from build123d import *

# Parameters (mm, degrees)
SKETCH1_R                           = 5
BOSS_EXTRUDE1_DEPTH                 = 403.4811
CHAMFER1_SIZE                       = 0.5
M5X0_8_TAPPED_HOLE1_D               = 4.2
M5X0_8_TAPPED_HOLE1_DEPTH           = 16.4
M5X0_8_TAPPED_HOLE1_TIP             = 1.2618073
M5X0_8_TAPPED_HOLE1_ON_FACE_2_D     = 4.2
M5X0_8_TAPPED_HOLE1_ON_FACE_2_DEPTH = 16.4
M5X0_8_TAPPED_HOLE1_ON_FACE_2_TIP   = 1.2618073


with BuildPart() as part:
    # Sketch1 → Boss-Extrude1 (new body)
    with BuildSketch(Plane.XY):
        Circle(SKETCH1_R)
    extrude(amount=BOSS_EXTRUDE1_DEPTH)

    # Chamfer1
    chamfer1_edges = [part.edges().sort_by_distance(p)[0] for p in [
        (-5, 0, 0),
        (-5, 0, 403.4811),
    ]]
    chamfer(chamfer1_edges, length=CHAMFER1_SIZE)

    # M5x0.8 Tapped Hole1
    with Locations(Plane.XY.offset(403.4811)):
        with Locations((0, 0)):
            Hole(M5X0_8_TAPPED_HOLE1_D / 2, depth=M5X0_8_TAPPED_HOLE1_DEPTH)
            with Locations((0, 0, -(M5X0_8_TAPPED_HOLE1_DEPTH + M5X0_8_TAPPED_HOLE1_TIP / 2))):  # 118° drill point
                Cone(0, M5X0_8_TAPPED_HOLE1_D / 2, M5X0_8_TAPPED_HOLE1_TIP, mode=Mode.SUBTRACT)

    # M5x0.8 Tapped Hole1 on face 2
    with Locations(Plane(origin=(0, 0, 0), x_dir=(-1, 0, 0), z_dir=(0, 0, -1))):
        with Locations((0, 0)):
            Hole(M5X0_8_TAPPED_HOLE1_ON_FACE_2_D / 2, depth=M5X0_8_TAPPED_HOLE1_ON_FACE_2_DEPTH)
            with Locations((0, 0, -(M5X0_8_TAPPED_HOLE1_ON_FACE_2_DEPTH + M5X0_8_TAPPED_HOLE1_ON_FACE_2_TIP / 2))):  # 118° drill point
                Cone(0, M5X0_8_TAPPED_HOLE1_ON_FACE_2_D / 2, M5X0_8_TAPPED_HOLE1_ON_FACE_2_TIP, mode=Mode.SUBTRACT)


solid = part.part
Geometry: final body of the model. Coordinates: model frame, mm. Give positions to 0.01 mm unless a question says otherwise; leave off trailing zeros. Order: outer loops, then holes, each group sorted by start corner. A loop starts at its lowest first (then second) coordinate and runs counter-clockwise, first axis right, second up. Notation, with made-up numbers: (59.5, 87.25) -> (108.5, 87.25) arc R22 ccw to (108.5, 96.25) -> close; hole circle Ø6 at (65.5, 10.5). An arc over 180 degrees is marked (long way). Answer as a JSON object with one key per item and string values.
Q1. Material intervals for probe 1 along Y at (x, z) = (0, 7.25); probe 2 along Y at (x, z) = (-0.25, 210); probe 3 along X at (y, z) = (-0.5, 143), sorted ascending.
Entries:
{"probe 1": "y = -5 to -2.1, 2.1 to 5", "probe 2": "y = -4.99 to 4.99", "probe 3": "x = -4.97 to 4.97"}
Q2. Section A-A (z = 120). Output: boundary loops of the cut face in (x, y), plus the area to 3 significant figures.
Entries:
{"outline": "circle Ø10 at (0, 0)", "area": "78.5 mm^2"}
Q3. First-contact query: pin 1 (1 mm diameter, centred on y = 1, z = 97.5, fed in from +X); pin 2 (2.5 mm diameter, centred on x = 0, y = 0, fed in from -Z). Flat tips, straight axial feed; report the tip coordinate or a pass-through.
Entries:
{"pin 1": "stops at x = 4.97", "pin 2": "stops at z = 16.91"}
